from build123d import *

# Parameters (mm, degrees)
F0_W     = 120.65
F0_H     = 44.45
F1_DEPTH = 66.675
F2_W     = 95.25
F2_H     = 25.4
F3_DEPTH = 66.676
F4_W     = 57.15
F4_H     = 15.875
F5_DEPTH = 19.051
F7_DEPTH = 19.051
F9_DEPTH = 25.401


with BuildPart() as f1:
    # F0 (on Front) → F1 (new body)
    with BuildSketch(Plane.XZ):
        with Locations((-4.2862482369, -12.2960915925)):
            Rectangle(F0_W, F0_H)
    extrude(amount=-F1_DEPTH)

    # F2 (on face) → F3 (cut, through all)
    with BuildSketch(Plane.XZ):
        with Locations((8.4137517631, -2.7710915925)):
            Rectangle(F2_W, F2_H)
    extrude(amount=-F3_DEPTH, mode=Mode.SUBTRACT)

    # F4 (on face) → F5 (cut, through all)
    with BuildSketch(Plane.XY.offset(-15.4710915925)):
        with Locations((27.4637517631, 33.3375)):
            Rectangle(F4_W, F4_H)
    extrude(amount=-F5_DEPTH, mode=Mode.SUBTRACT)

    # F6 (on face) → F7 (cut, through all)
    with BuildSketch(Plane.XY.offset(-15.4710915925)):
        Polygon((56.0387517631, 66.675), (24.2887517631, 66.675), (56.0387517631, 48.3441289532), align=None)
        Polygon((56.0387517631, 0), (56.0387517631, 18.3308710468), (24.2887517631, 0), align=None)
    extrude(amount=-F7_DEPTH, mode=Mode.SUBTRACT)

    # F8 (on face) → F9 (cut, through all)
    with BuildSketch(Plane.YZ.offset(-39.2112482369)):
        Polygon((19.05, 9.9289084075), (11.7176515813, -2.7710915925), (54.9573484187, -2.7710915925), (47.625, 9.9289084075), align=None)
    extrude(amount=-F9_DEPTH, mode=Mode.SUBTRACT)


solid = f1.part
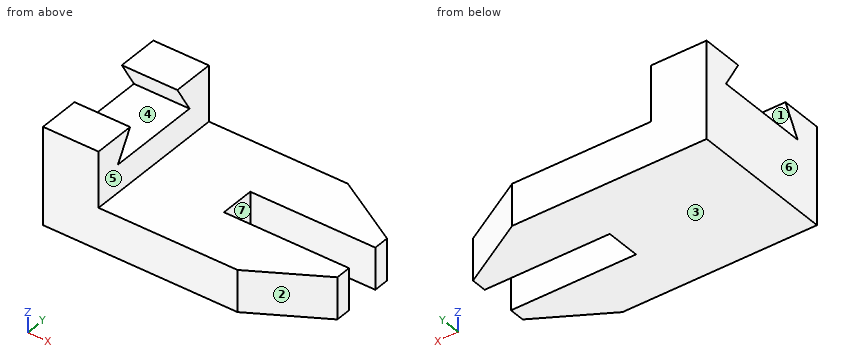
CAD build for the part. Positions are in the model's coordinates, mm. Face numbers are marked on the shaded views. A direction names the side the tool comes from. Coordinates: 2 decimals unless noted, no trailing zeros. Order: outer loops, then holes, each group sorted by start corner. A loop starts at its lowest first (then second) coordinate and runs counter-clockwise, first axis right, second up. Notation, with made-up numbers: (26.5, -3) -> (50.5, -3) arc R22 ccw to (50.5, 13) -> close; hole circle Ø2 at (21.5, 4). An arc over 180 degrees is marked (long way). Answer in a Markdown table with one row per item.
1) Band-saw the part on A-A (x = 20). List the corners of the cut face in (y, z) (3 decimals).
Check values:
| item | result |
|---|---|
| outline | (0, -34.521) -> (25.4, -34.521) -> (25.4, -15.471) -> (0, -15.471) -> close; (41.275, -34.521) -> (66.675, -34.521) -> (66.675, -15.471) -> (41.275, -15.471) -> close |
2) Band-saw the part on D-D (x = -44). List the corners of the cut face in (y, z) (3 decimals), and give its area (3 significant figures).
Check values:
| item | result |
|---|---|
| outline | (0, -34.521) -> (66.675, -34.521) -> (66.675, 9.929) -> (47.625, 9.929) -> (54.957, -2.771) -> (11.718, -2.771) -> (19.05, 9.929) -> (0, 9.929) -> close |
| area | 2,510 mm2 |
3) Mould opens along Z. For the marked faces 1, 2, 3 and 4 say: pulls with the +Z half, pulls with the -Z half, needs draft (parallel to the pull), parting line crosses it, or undercut.
Check values:
| item | result |
|---|---|
| face 1 | undercut |
| face 2 | needs draft |
| face 3 | pulls with the -Z half |
| face 4 | undercut |
4) Which spindle directions (+Z, -Z, +X, -X, +Y, -Y) get a long thin tool onto all of the face, cutting with end or side? Do the marked faces 5, 6 and 7. Say none if no direction does.
Check values:
| item | result |
|---|---|
| face 5 | +Z, +X, +Y, -Y |
| face 6 | +Z, -Z, -X, +Y, -Y |
| face 7 | +Z, -Z, +X |
5) Band-saw the part on C-C (z = 5). List the corners of the cut face in (x, y) (3 decimals), and give its area (3 significant figures).
Check values:
| item | result |
|---|---|
| outline | (-64.611, 0) -> (-39.211, 0) -> (-39.211, 16.204) -> (-64.611, 16.204) -> close; (-64.611, 50.471) -> (-39.211, 50.471) -> (-39.211, 66.675) -> (-64.611, 66.675) -> close |
| area | 823 mm2 |
6) Drill centre lines: line 1 (Z direction, x = 26, y = 21); line 2 (X direction, y = 30.5, z = -22); line 3 (X direction, y = 59.5, z = -4). Where is each one in solid material? Low to high.
Check values:
| item | result |
|---|---|
| line 1 | -34.52 to -15.47 |
| line 2 | -64.61 to -1.11 |
| line 3 | -64.61 to -39.21 |
7) Flat gauge pins, fed straight in: P1, Ø8, axis at y = 29.5, z = -24, coming from the +X side; P2, Ø10, axis at y = 52, z = 2.5, coming from the +X side; P3, Ø7.5, axis at x = -47.5, y = 30.5, coming from the +Z side. Where does each tip first touch, or does it go through?
Check values:
| item | result |
|---|---|
| P1 | x = -1.11 |
| P2 | x = -39.21 |
| P3 | z = -2.77 |
8) Band-saw the part on B-B (y = 51). List the corners of the cut face in (x, z), and give its area (3 significant figures).
Check values:
| item | result |
|---|---|
| outline | (-64.61, -34.52) -> (51.44, -34.52) -> (51.44, -15.47) -> (-39.21, -15.47) -> (-39.21, -2.77) -> (-64.61, -2.77) -> close; (-64.61, 4.08) -> (-39.21, 4.08) -> (-39.21, 9.93) -> (-64.61, 9.93) -> close |
| area | 2,680 mm2 |
